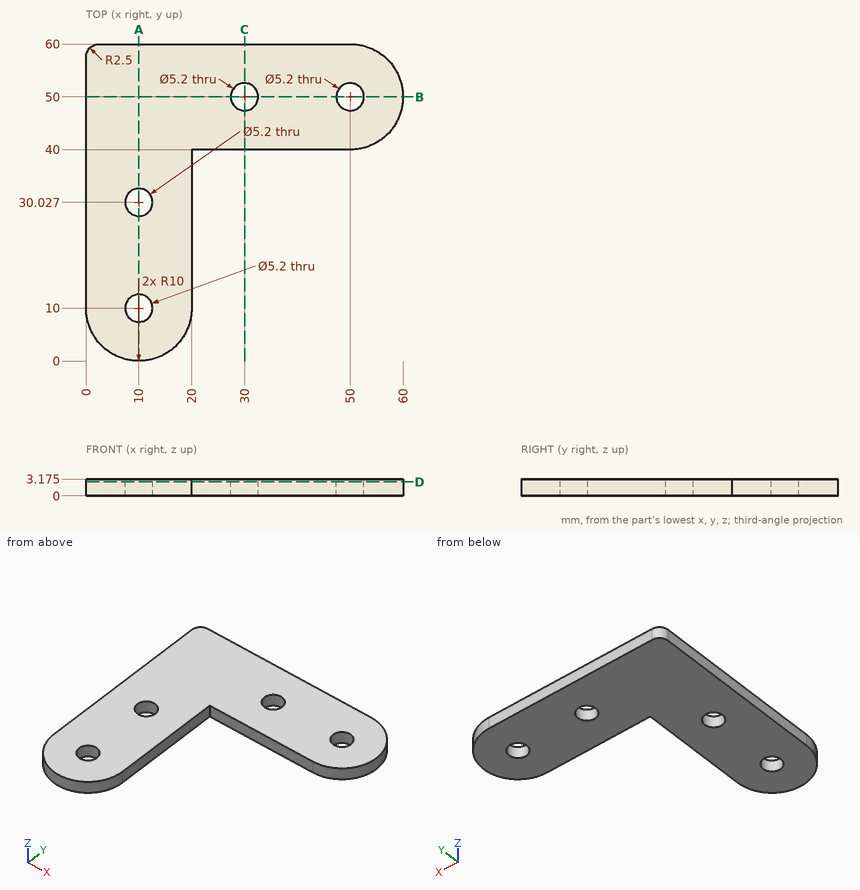
Design review of the part shown in the three views and the two pictorial views. Dimensions are in mm from the part's minimum x, y and z. Round coordinates to 2 decimals unless told otherwise and drop trailing zeros. Loops run counter-clockwise (first coordinate to the right, second up) from the corner with the lowest first, then second, coordinate; pieces in that order, holes last. Notation, with made-up numbers: (56.5, 17.25) -> (61.5, 17.25) arc R7 ccw to (61.5, 25.25) -> close; hole circle Ø11 at (45.5, -30). An arc over 180 degrees is marked (long way). Use one line per item in the form item = value. Start each with the question number.
Q1. For pin 1 Ø1 at (x, z) = (35, 1) entering from -Y, flat-tipped, find the tip position at first contact; note if it passes through.
Q2. Wall thickness on line 1 along Y through (x, z) = (10, 1.1); line 2 along Y through (x, z) = (12, 1.75) (1 decimal); line 3 along X through (y, z) = (16, 0.35): over which ranges is each line inside the solid? List them lowest first. Write a range as [from, to].
Q3. We need section C-C on x = 30. Give the boundary of the cut face in (y, z) (3 decimals).
Q4. We need section D-D on z = 2.65. Give the boundary of the cut face in (x, y), then the cut area to 3 significant figures.
Q5. We need section B-B on y = 50. Give the boundary of the cut face in (x, z) (3 decimals).
Q6. We need section A-A on x = 10. Give the boundary of the cut face in (y, z) (3 decimals), then the cut area to 4 significant figures.
Calculated:
q1.pin_1 = 40
q2.line_1 = [0, 7.4], [12.6, 27.43], [32.63, 60]
q2.line_2 = [0.2, 8.3], [11.7, 28.4], [31.7, 60]
q2.line_3 = [0, 20]
q3.outline = (40, 0) -> (47.4, 0) -> (47.4, 3.175) -> (40, 3.175) -> close; (52.6, 0) -> (60, 0) -> (60, 3.175) -> (52.6, 3.175) -> close
q4.outline = (0, 10) arc R10 ccw to (20, 10) -> (20, 40) -> (50, 40) arc R10 ccw to (50, 60) -> (2.5, 60) arc R2.5 ccw to (0, 57.5) -> close; hole circle Ø5.2 at (10, 10); hole circle Ø5.2 at (10, 30.03); hole circle Ø5.2 at (30, 50); hole circle Ø5.2 at (50, 50)
q4.area = 1,830 mm²
q5.outline = (0, 0) -> (27.4, 0) -> (27.4, 3.175) -> (0, 3.175) -> close; (32.6, 0) -> (47.4, 0) -> (47.4, 3.175) -> (32.6, 3.175) -> close; (52.6, 0) -> (60, 0) -> (60, 3.175) -> (52.6, 3.175) -> close
q6.outline = (0, 0) -> (7.4, 0) -> (7.4, 3.175) -> (0, 3.175) -> close; (12.6, 0) -> (27.427, 0) -> (27.427, 3.175) -> (12.6, 3.175) -> close; (32.627, 0) -> (60, 0) -> (60, 3.175) -> (32.627, 3.175) -> close
q6.area = 157.5 mm²
